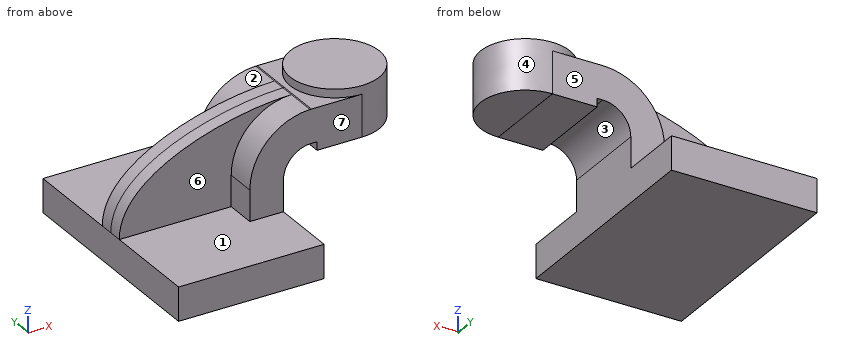
from build123d import *

# Parameters (mm, degrees)
F1_DEPTH = 63.5
F2_DEPTH = 25.4
F3_DEPTH = 25.4
F4_DEPTH = 7.9375


with BuildPart() as f1:
    # F0 (on Front) → F1 (new body, symmetric)
    with BuildSketch(Plane.XZ):
        Polygon((23.747439423, 9.525), (-39.752560577, 9.525), (-39.752560577, -9.525), (42.797439423, -9.525), (42.797439423, 9.525), align=None)
    extrude(amount=F1_DEPTH, both=True)

    # F0 (on Front) → F2 (join, symmetric)
    with BuildSketch(Plane.XZ):
        with BuildLine():
            Line((23.747439423, 27.0002), (23.747439423, 9.525))
            Line((23.747439423, 9.525), (42.797439423, 9.525))
            Line((42.797439423, 9.525), (42.797439423, 27.0002))
            ThreePointArc((42.797439423, 27.0002), (47.4471192717, 38.2255201513), (58.672439423, 42.8752))
            Line((58.672439423, 42.8752), (61.847439423, 42.8752))
            Line((61.847439423, 42.8752), (61.847439423, 61.9252))
            Line((61.847439423, 61.9252), (58.672439423, 61.9252))
            add(Edge.make_bspline(
                [(57.9305268727, 61.9173188784), (58.1788443539, 61.9206892677), (58.4261566277, 61.9233163085), (58.672439423, 61.9252)],
                knots=[110.7711022014, 110.7711022014, 110.7711022014, 110.7711022014, 111.5045361635, 111.5045361635, 111.5045361635, 111.5045361635], degree=3))
            ThreePointArc((57.9305268727, 61.9173188784), (33.7158078312, 51.4321905982), (23.747439423, 27.0002))
        make_face()
    extrude(amount=F2_DEPTH, both=True)

    # F0 (on Front) → F3 (join, symmetric)
    with BuildSketch(Plane.XZ):
        Polygon((87.2794313061, 61.9252), (61.847439423, 61.9252), (61.847439423, 42.8752), (61.847439423, 38.1), (87.247439423, 38.1), align=None)
    extrude(amount=F3_DEPTH, both=True)

    # F0 (on Front) → F4 (join, symmetric)
    with BuildSketch(Plane.XZ):
        with BuildLine():
            add(Edge.make_bspline(
                [(-39.752560577, 9.525), (-40.0057176122, 43.9432543149), (20.4269443953, 61.4082863569), (57.9305268727, 61.9173188784)],
                knots=[0, 0, 0, 0, 110.7711022014, 110.7711022014, 110.7711022014, 110.7711022014], degree=3))
            Line((-39.752560577, 9.525), (23.747439423, 9.525))
            Line((23.747439423, 9.525), (23.747439423, 27.0002))
            ThreePointArc((23.747439423, 27.0002), (33.7158078312, 51.4321905982), (57.9305268727, 61.9173188784))
        make_face()
    extrude(amount=F4_DEPTH, both=True)

    # F0 (on Front) → F5 (revolve)
    with BuildSketch(Plane.XZ):
        Polygon((87.2858092189, 66.675), (87.2794313061, 61.9252), (87.247439423, 38.1), (112.647439423, 38.1), (112.647439423, 66.675), align=None)
    revolve(axis=Axis((87.2666243209, 0, 52.3875), (0.0013427738, 0, 0.9999990985)))


solid = f1.part
Read the model definition and answer for the solid it produces. Units are mm, in the model's axes. Face numbers are marked on the shaded views. A direction names the side the tool comes from. Round coordinates to 2 decimals unless told otherwise and drop trailing zeros. Loops run counter-clockwise (first coordinate to the right, second up) from the corner with the lowest first, then second, coordinate; pieces in that order, holes last.
Q1. Determine the mould class of the marked faces 1, 2, 3 and 4 for opening direction X: released by +X, released by -X, zero draft, split by the parting line, or undercut.
Q2. Which of the six approach directions +Z, -Z, +X, -X, +Y, -Y give full straight-line access (tool end or side, diameter ignored) to the marked faces 5, 6 and 7?
Q3. Each of these flat-tipped pins is pushed along its axis until it touches: pin 1 (12 mm diameter, centred on x = 16.5, z = 39, fed in from -Y); pin 2 (23 mm diameter, centred on x = 76.5, y = 11.5, fed in from +Z); pin 3 (15.5 mm diameter, centred on x = 26, z = 47, fed in from -Y). Where does it stop, or does it pass through?
Q4. Consider probe 1 along Z at (x, y) = (12, -39.5) (3 decimals); probe 2 along Y at (x, z) = (-14, 21); probe 3 along X at (y, z) = (-0.5, 11). Determine where each line is inside the solid, lowest interval first.
Q5. Section A-A on y = 54 is taken. Write down the section's boundary in (x, z) (3 decimals), and give its area (3 significant figures).
Q6. Section B-B on z = 3 is taken. Write down the section's boundary in (x, y), and give its area (3 significant figures).
Output:
1. face 1: zero draft
1. face 2: released by -X
1. face 3: undercut
1. face 4: split by the parting line
2. face 5: +Z, +X, -X, +Y
2. face 6: +Z, -X, -Y
2. face 7: +Z, +X, -X, -Y
3. pin 1: stops at y = -7.94
3. pin 2: stops at z = 66.74
3. pin 3: stops at y = -25.4
4. probe 1: z = -9.525 to 9.525
4. probe 2: y = -7.94 to 7.94
4. probe 3: x = -39.73 to 42.8
5. outline: (-39.753, -9.525) - (42.797, -9.525) - (42.797, 9.525) - (-39.753, 9.525) - close
5. area: 1,570 mm2
6. outline: (-39.75, -63.5) - (42.8, -63.5) - (42.8, 63.5) - (-39.75, 63.5) - close
6. area: 10,500 mm2
